from build123d import *

# Parameters (mm, degrees)
SKETCH3_W           = 0.381
SKETCH3_H           = 0.381
BOSS_EXTRUDE1_DEPTH = 5.08
SKETCH3_4_W         = 0.381
SKETCH3_4_H         = 0.381
BOSS_EXTRUDE2_DEPTH = 2.54
ECHELLE1_SCALE      = 4


with BuildPart() as part:
    # Sketch2 → Revolve1 (revolve)
    with BuildSketch(Plane.XY, mode=Mode.PRIVATE) as revolve1_sk:
        with BuildLine():
            Line((0, 0), (2.794, 0))
            Line((2.794, 0), (2.794, 1.143))
            Line((2.794, 1.143), (2.3495, 1.143))
            Line((2.3495, 1.143), (2.3495, 6.3881))
            ThreePointArc((2.3495, 6.3881), (1.661347382, 8.049447382), (0, 8.7376))
            Line((0, 8.7376), (0, 0))
        make_face()
    revolve(revolve1_sk.sketch.rotate(Axis((0, 0, 0), (0, 1, 0)), 90), axis=Axis((0, 0, 0), (0, 1, 0)))

    # Sketch3 → Boss-Extrude1 (add)
    with BuildSketch(Plane.XZ):
        with Locations((0.9525, 0)):
            Rectangle(SKETCH3_W, SKETCH3_H)
    extrude(amount=BOSS_EXTRUDE1_DEPTH)

    # Sketch3_4 → Boss-Extrude2 (add)
    with BuildSketch(Plane.XZ):
        with Locations((-0.9525, 0)):
            Rectangle(SKETCH3_4_W, SKETCH3_4_H)
    extrude(amount=BOSS_EXTRUDE2_DEPTH)


with BuildPart() as part_1:
    # Echelle1: scaled about (0.002384831, 3.75963667, 0)
    add(part.part.scale(ECHELLE1_SCALE).moved(Location((-0.007154493, -11.27891001, 0))))


solid = part_1.part
CAD build for the part. Positions are in the model's coordinates, mm. A direction names the side the tool comes from. Coordinates: 2 decimals unless noted, no trailing zeros. Order: outer loops, then holes, each group sorted by start corner. A loop starts at its lowest first (then second) coordinate and runs counter-clockwise, first axis right, second up. Notation, with made-up numbers: (-17, -9) -> (33, -9) arc R22 ccw to (33, 9) -> close; hole circle Ø11 at (53, 11.5). An arc over 180 degrees is marked (long way). Answer in a Markdown table with one row per item.
1) Band-saw the part on C-C (x = -7.75). List the corners of the cut face in (y, z).
Check values:
| item | result |
|---|---|
| outline | (-11.28, -8.06) -> (-6.71, -8.06) -> (-6.71, -5.33) -> (14.27, -5.33) arc R5.33 ccw to (14.27, 5.33) -> (-6.71, 5.33) -> (-6.71, 8.06) -> (-11.28, 8.06) -> close |
2) Band-saw the part on B-B (z = 0). List the corners of the cut face in (x, y).
Check values:
| item | result |
|---|---|
| outline | (-11.18, -11.28) -> (-4.58, -11.28) -> (-4.58, -21.44) -> (-3.06, -21.44) -> (-3.06, -11.28) -> (3.04, -11.28) -> (3.04, -31.6) -> (4.56, -31.6) -> (4.56, -11.28) -> (11.17, -11.28) -> (11.17, -6.71) -> (9.39, -6.71) -> (9.39, 14.27) arc R9.4 ccw to (-9.41, 14.27) -> (-9.41, -6.71) -> (-11.18, -6.71) -> close |
3) Which spindle directions (+Z, -Z, +X, -X, +Y, -Y) get a long thin tool onto all of the face, cutting with end or side? Do faces 1 (the face through (-4, -21.439, 0)), 2 (the face through (-9.325, 3.93, 1.223)), 3 (the face through (4, -21, -0.762)), 4 (the face through (3.041, -21, 0)), 5 (the face through (4, -21, 0.762)). Say none if no direction does.
Check values:
| item | result |
|---|---|
| face 1 | +Z, -Z, -X, -Y |
| face 2 | +Y |
| face 3 | -Z, +X, -X, -Y |
| face 4 | +Z, -Z, -Y |
| face 5 | +Z, +X, -X, -Y |
4) Drill centre lines: line 1 (Y direction, x = -10.5, z = 0.75); line 2 (X direction, y = 14.5, z = 0); line 3 (Z direction, x = -4.5, y = -14). Where is each one in solid material? Low to high.
Check values:
| item | result |
|---|---|
| line 1 | -11.28 to -6.71 |
| line 2 | -9.4 to 9.39 |
| line 3 | -0.76 to 0.76 |
5) Flat gauge pins, fed straight in: P1, Ø2, axis at y = 7.5, z = 1.5, coming from the -X side; P2, Ø1.2, axis at x = 4, y = -20.5, coming from the -Z side; P3, Ø2, axis at x = -8, z = -1, coming from the +Y side. Where does each tip first touch, or does it go through?
Check values:
| item | result |
|---|---|
| P1 | x = -9.39 |
| P2 | z = -0.76 |
| P3 | y = 20.48 |
6) Band-saw the part on A-A (y = -19). List the corners of the cut face in (x, z), and give its area (3 significant figures).
Check values:
| item | result |
|---|---|
| outline | (-4.58, -0.76) -> (-3.06, -0.76) -> (-3.06, 0.76) -> (-4.58, 0.76) -> close; (3.04, -0.76) -> (4.56, -0.76) -> (4.56, 0.76) -> (3.04, 0.76) -> close |
| area | 4.65 mm2 |
7) Band-saw the part on D-D (y = -27.5). List the corners of the cut face in (x, z), and give its area (3 significant figures).
Check values:
| item | result |
|---|---|
| outline | (3.04, -0.76) -> (4.56, -0.76) -> (4.56, 0.76) -> (3.04, 0.76) -> close |
| area | 2.32 mm2 |
